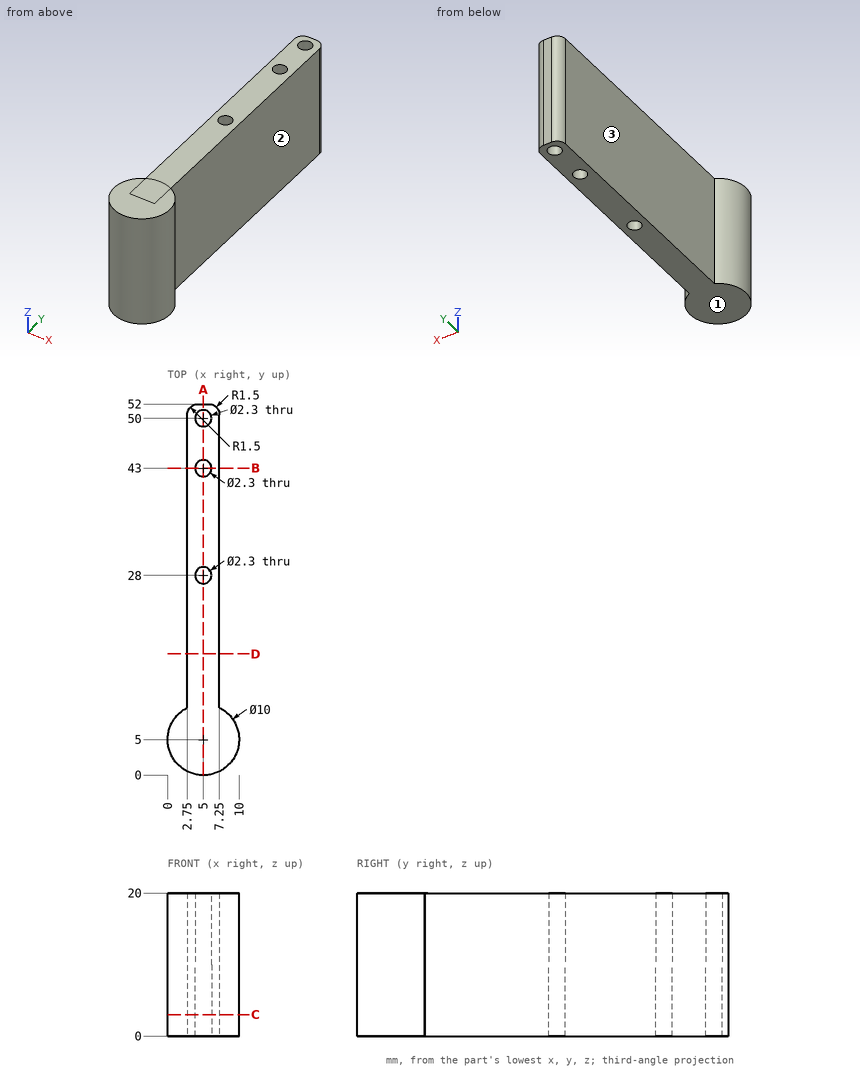
Verification items for this drawing (mm, ordinates from the low corner). A direction names the side the tool comes from. Round coordinates to 2 decimals unless told otherwise and drop trailing zeros. Order: outer loops, then holes, each group sorted by start corner. A loop starts at its lowest first (then second) coordinate and runs counter-clockwise, first axis right, second up. Notation, with made-up numbers: (-28.5, -3) - (-11.5, -3) arc R25 ccw to (-11.5, 14) - close; hole circle Ø3 at (77, 6). An arc over 180 degrees is marked (long way). Use CSV: the item, a comma, the result in double quotes. Start each with the question number.
1) Thickness scan on L1, parallel to Y at x = 5, z = 16; L2, parallel to Y at x = 5.5, z = 19.25; L3, parallel to X at y = 43, z = 4.5. Record the ranges inside material, lowest first.
2) Section check A-A, the plane x = 5. Record the cut outline in (y, z).
3) Go/stop test with flat-tipped pins: P1, Ø1, axis at y = 8.5, z = 12.5, coming from the -X side; P2, Ø1.5, axis at x = 1.5, z = 8, coming from the -Y side; P3, Ø8, axis at y = 33.5, z = 17, coming from the -X side; P4, Ø1.8, axis at x = 5, y = 50, coming from the +Z side. Record where each tip stops, or that it passes through.
4) Access from +Z, -Z, +X, -X, +Y, -Y to the whole of each face (thin tool, end or side, straight path). Record for the marked faces 1, 2 and 3.
5) Section check B-B, the plane y = 43. Record the cut outline in (x, z), plus the area to 3 significant figures.
6) Section check C-C, the plane z = 3. Record the cut outline in (x, y), plus the area to 3 significant figures.
7) Section check D-D, the plane y = 17. Record the cut outline in (x, z).
Answers:
1,L1,"y = 0 to 26.85, 29.15 to 41.85, 44.15 to 48.85, 51.15 to 52"
1,L2,"y = 0.03 to 26.96, 29.04 to 41.96, 44.04 to 48.96, 51.04 to 52"
1,L3,"x = 2.75 to 3.85, 6.15 to 7.25"
2,outline,"(0, 0) - (26.85, 0) - (26.85, 20) - (0, 20) - close; (29.15, 0) - (41.85, 0) - (41.85, 20) - (29.15, 20) - close; (44.15, 0) - (48.85, 0) - (48.85, 20) - (44.15, 20) - close; (51.15, 0) - (52, 0) - (52, 20) - (51.15, 20) - close"
3,P1,"stops at x = 1"
3,P2,"stops at y = 0.82"
3,P3,"stops at x = 2.75"
3,P4,"passes through"
4,face 1,"-Z, +X, -X, +Y, -Y"
4,face 2,"+Z, -Z, +X, +Y"
4,face 3,"+Z, -Z, -X, +Y"
5,outline,"(2.75, 0) - (3.85, 0) - (3.85, 20) - (2.75, 20) - close; (6.15, 0) - (7.25, 0) - (7.25, 20) - (6.15, 20) - close"
5,area,"44.0 mm²"
6,outline,"(2.75, 9.47) arc R5 ccw (long way) to (7.25, 9.47) - (7.25, 50.5) arc R1.5 ccw to (5.75, 52) - (4.25, 52) arc R1.5 ccw to (2.75, 50.5) - close; hole circle Ø2.3 at (5, 28); hole circle Ø2.3 at (5, 43); hole circle Ø2.3 at (5, 50)"
6,area,"255 mm²"
7,outline,"(2.75, 0) - (7.25, 0) - (7.25, 20) - (2.75, 20) - close"
